Autodesk Inventor part; units mm, degrees
ref_plane "YZ Plane" through (0, 0, 0) normal (1, 0, 0) x (0, 1, 0)
ref_plane "XZ Plane" through (0, 0, 0) normal (0, 1, 0) x (-1, 0, 0)
ref_plane "XY Plane" through (0, 0, 0) normal (0, 0, 1) x (1, 0, 0)
sketch "CONTOURS" plane through (0, 0, 0) normal (0, 0, 1) x (1, 0, 0)
  line L0 (25, 917.9541) -> (25, 902.2281)
  arc A0 (25, 902.2281) -> (27, 900.2277) centre (27, 902.2277) ccw
  line L1 (27, 900.2277) -> (143, 900.2277)
  arc A1 (143, 900.2277) -> (145, 902.2277) centre (143, 902.2277) ccw
  line L2 (145, 902.2277) -> (145, 908.2874)
  arc A2 (145, 908.2874) -> (143.1661, 910.2805) centre (143, 908.2874) ccw
  line L3 (143.1661, 910.2805) -> (27.1661, 919.9472)
  arc A3 (27.1661, 919.9472) -> (25, 917.9541) centre (27, 917.9541) ccw
extrude "Extrusion1" add sketch "CONTOURS" along normal blind 18
properties part number "Wedge" material "Wood (Birch)"
Check sheet for the modelled part. Datum: model origin and axes. Units: mm. Give positions to 0.01 mm unless a question says otherwise; leave off trailing zeros. Write each loop counter-clockwise with the first axis right and the second up, starting at its lowest first coordinate (ties: lowest second). Pieces come first, ordered by that corner, then holes.
Item 1: Cross-section at B-B (y = 915). Enter the section's corners in (x, z).
Item 2: Scan lines: L1, parallel to Y at x = 82.5, z = 3.5; L2, parallel to Y at x = 68, z = 7.5; L3, parallel to X at y = 908.75, z = 13.75. Record each from-to range of solid material in increasing order.
Item 3: Cross-section at C-C (x = 109.5). Enter the section's corners in (y, z), and give its area (3 significant figures).
Item 4: Cross-section at A-A (z = 6). Enter the section's corners in (x, y), and give its area (3 significant figures).
Item 5: Draft check along Z on faces 1 (the face through (84, 908, 0)), 2 (the face through (144.458, 909.657, 8.874)), 3 (the face through (84, 908, 18)). Enter one of: released by +Z, released by -Z, zero draft, split by the parting line, or undercut.
Report:
1. outline: (25, 0) - (86.53, 0) - (86.53, 18) - (25, 18) - close
2. L1: y = 900.23 to 915.34
2. L2: y = 900.23 to 916.54
2. L3: x = 25 to 144.95
3. outline: (900.23, 0) - (913.09, 0) - (913.09, 18) - (900.23, 18) - close
3. area: 231 mm2
4. outline: (25, 902.23) arc R2 ccw to (27, 900.23) - (143, 900.23) arc R2 ccw to (145, 902.23) - (145, 908.29) arc R2 ccw to (143.17, 910.28) - (27.17, 919.95) arc R2 ccw to (25, 917.95) - close
4. area: 1,780 mm2
5. face 1: released by -Z
5. face 2: zero draft
5. face 3: released by +Z
